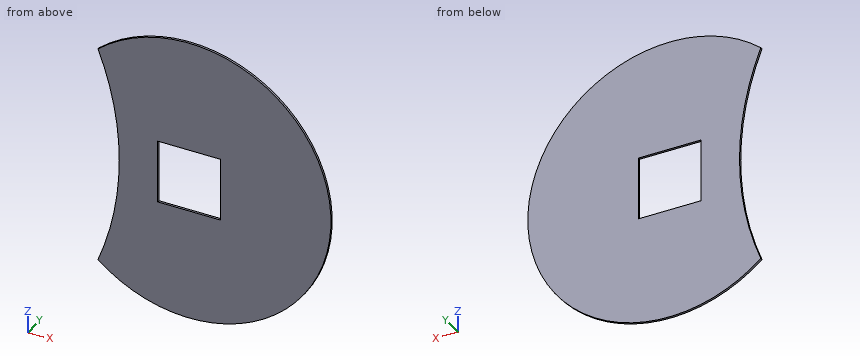
from build123d import *

# Parameters (mm, degrees)
F0_R     = 190
F1_DEPTH = 3
F2_W     = 42
F2_H     = 42
F3_DEPTH = 3.001
F5_DEPTH = 3.001


with BuildPart() as f1:
    # F0 (on Front) → F1 (new body)
    with BuildSketch(Plane.XZ):
        Circle(F0_R)
    extrude(amount=F1_DEPTH)

    # F2 (on face) → F3 (cut, through all)
    with BuildSketch(Plane.XZ.offset(3)):
        with Locations((-21, -21)):
            Rectangle(F2_W, F2_H)
        with Locations((21, -21)):
            Rectangle(F2_W, F2_H)
        with Locations((21, 21)):
            Rectangle(F2_W, F2_H)
        with Locations((-21, 21)):
            Rectangle(F2_W, F2_H)
    extrude(amount=-F3_DEPTH, mode=Mode.SUBTRACT)

    # F4 (on face) → F5 (cut, through all)
    with BuildSketch(Plane.XZ.offset(3)):
        with BuildLine():
            ThreePointArc((-122, -145.6571316483), (-100.6859205662, -74.2103602534), (-93.4919261309, 0))
            Line((-93.4919261309, 0), (-122, 0))
            Line((-122, 0), (-122, -145.6571316483))
        make_face()
        with BuildLine():
            Line((-122, 0), (-93.4919261309, 0))
            ThreePointArc((-93.4919261309, 0), (-100.6859205662, 74.2103602533), (-122, 145.6571316483))
            Line((-122, 145.6571316483), (-122, 0))
        make_face()
        with BuildLine():
            Line((-122, -145.6571316483), (-122, 0))
            Line((-122, 0), (-122, 145.6571316483))
            ThreePointArc((-122, 145.6571316483), (-190, 0), (-122, -145.6571316483))
        make_face()
    extrude(amount=-F5_DEPTH, mode=Mode.SUBTRACT)


solid = f1.part
Work out the finished part from the listing and answer in its coordinate system (mm). Give positions to 0.01 mm unless a question says otherwise; leave off trailing zeros. Loops run counter-clockwise (first coordinate to the right, second up) from the corner with the lowest first, then second, coordinate; pieces in that order, holes last. Notation, with made-up numbers: M 27.25,60 L 45.25,60 A30 cw 45.25,96 Z; hole C 25,77.25 d6. An arc over 180 degrees is marked long. Use CSV: the item, a comma, the result in double quotes.
1) Given P1, Ø1.5, axis at x = 19.5, y = -2, coming from the +Z side; P2, Ø1.5, axis at x = 20, y = -2, coming from the -Z side, each flat-ended and moving along its own axis, determine where each tip first touches the part or whether it passes through.
Answer:
P1,"z = 189.07"
P2,"z = -189.02"
2) Consider L1, parallel to Z at x = 2, y = -1.9; L2, parallel to Z at x = -9.5, y = -2.6; L3, parallel to X at y = -0.85, z = 39.5. Determine where each line is inside the solid, lowest interval first.
Answer:
L1,"-189.99 to -42, 42 to 189.99"
L2,"-189.76 to -42, 42 to 189.76"
L3,"-95.52 to -42, 42 to 185.85"
3) Find section A-A on x = 0. Write down the section's boundary in (y, z).
Answer:
outline,"M -3,-190 L 0,-190 L 0,-42 L -3,-42 Z; M -3,42 L 0,42 L 0,190 L -3,190 Z"
4) Find section B-B on y = -1.05. Write down the section's boundary in (x, z).
Answer:
outline,"M -122,-145.66 A190 ccw long -122,145.66 A386.36 cw Z; hole M -42,-42 L 42,-42 L 42,42 L -42,42 Z"
5) Find section D-D on z = -109.5. Write down the section's boundary in (x, y), plus the area to 3 significant figures.
Answer:
outline,"M -109.33,-3 L 155.27,-3 L 155.27,0 L -109.33,0 Z"
area,"794 mm^2"
6) Find section C-C on x = -65. Write down the section's boundary in (y, z), plus the area to 3 significant figures.
Answer:
outline,"M -3,-178.54 L 0,-178.54 L 0,178.54 L -3,178.54 Z"
area,"1,070 mm^2"
